For this review, take the finished solid that the model builds, in its own axes (mm). Face numbers are marked on the shaded views. Coordinates: 2 decimals unless noted, no trailing zeros.
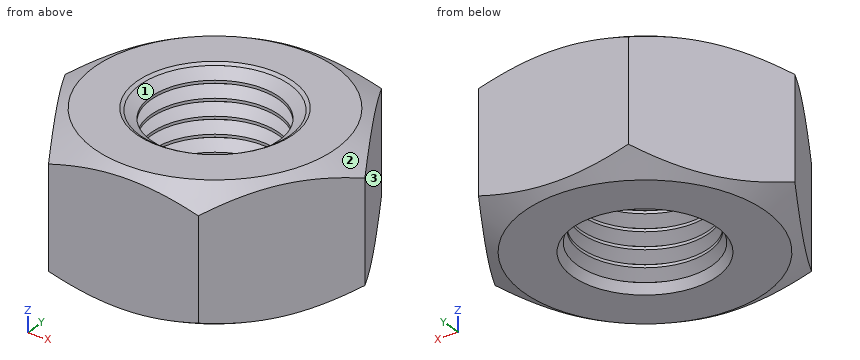
from build123d import *

# Parameters (mm, degrees)
SKETCH1_R               = 2.4585
BASENUT_DEPTH           = 5.2
ENDCHAMFER_SIZE         = 0.5415
ENDCHAMFER_SIZE2        = 0.312635171
ENDCHAMFER_PART_2_SIZE  = 0.5415
ENDCHAMFER_PART_2_SIZE2 = 0.312635171
LPATTERN10_COUNT        = 8
LPATTERN10_PITCH        = 0.6498


with BuildPart() as part:
    # Sketch1 → BaseNut (new body)
    with BuildSketch(Plane.XY):
        Polygon((5.773502692, 0), (2.886751346, 5), (-2.886751346, 5), (-5.773502692, 0), (-2.886751346, -5), (2.886751346, -5), align=None)
        Circle(SKETCH1_R, mode=Mode.SUBTRACT)
    extrude(amount=-BASENUT_DEPTH)

    # Sketch2 → Double-Chamfer (revolve, cut)
    with BuildSketch(Plane(origin=(0, 0, 0), x_dir=(1, 0, 0), z_dir=(0, 1, 0))):
        Polygon((-5.773502692, 5.2), (-4.625, 5.2), (-5.773502692, 4.536911662), align=None)
        Polygon((-5.773502692, 0.663088338), (-5.773502692, 0), (-4.625, 0), align=None)
    revolve(axis=Axis((0, 0, -3.375940562), (0, 0, 1)), mode=Mode.SUBTRACT)

    # EndChamfer
    endchamfer_edges = [part.edges().sort_by_distance(p)[0] for p in [
        (-2.4585, 0, -5.2),
    ]]
    endchamfer_side = [part.faces().sort_by_distance(p)[0] for p in [
        (-2.4585, 0, -2.6),
    ]]
    chamfer(endchamfer_edges, length=ENDCHAMFER_SIZE, length2=ENDCHAMFER_SIZE2, reference=endchamfer_side[0])

    # EndChamfer part 2
    endchamfer_part_2_edges = [part.edges().sort_by_distance(p)[0] for p in [
        (-2.4585, 0, 0),
    ]]
    endchamfer_part_2_side = [part.faces().sort_by_distance(p)[0] for p in [
        (4.494185245, 0, 0),
    ]]
    chamfer(endchamfer_part_2_edges, length=ENDCHAMFER_PART_2_SIZE, length2=ENDCHAMFER_PART_2_SIZE2, reference=endchamfer_part_2_side[0])

    # Sketch3 → Cut-Revolve10 (revolve, cut)
    with BuildSketch(Plane(origin=(0, 0, 0), x_dir=(1, 0, 0), z_dir=(0, 1, 0))):
        Polygon((-2.927452756, 4.6585), (-2.4585, 4.38775), (-1.917, 4.38775), (-1.917, 4.92925), (-2.4585, 4.92925), align=None)
    cut_revolve10 = revolve(axis=Axis((0, 0, -7.438254559), (0, 0, -1)), mode=Mode.SUBTRACT)

    # LPattern10: Cut-Revolve10 ×8
    with Locations(*[(0, 0, i * LPATTERN10_PITCH) for i in range(1, LPATTERN10_COUNT)]):
        add(cut_revolve10, mode=Mode.SUBTRACT)


solid = part.part
1. To check wall thickness, follow L1, parallel to Y at x = 0, z = -3; L2, parallel to X at y = 0.25, z = -5; L3, parallel to Y at x = 2, z = -2.4. State the ranges of each line that lie inside material, in increasing order.
Answer below:
L1: y = -5 to -2.46, 2.46 to 5
L2: x = -4.97 to -2.64, 2.64 to 4.97
L3: y = -5 to -1.43, 1.43 to 5
2. The part is to be moulded in two halves that separate along X. For the marked faces 1, 2 and 3, say which applies: +X half, -X half, draft (parallel to the pull), parting line (faces both ways), or undercut.
Answer below:
face 1: undercut
face 2: parting line
face 3: +X half
3. Clearance check with flat-ended pins moving along their axes: pin 1 Ø1 at (x, y) = (-2, -2) entering from +Z; pin 2 Ø5.5 at (x, y) = (0, 0) entering from +Z; pin 3 Ø2 at (y, z) = (-3.5, -4.5) entering from -X; pin 4 Ø2 at (y, z) = (2, -2.5) entering from +X. State where each tip first meets the part, or that it passes through.
Answer below:
pin 1: stops at z = 0
pin 2: stops at z = -0.21
pin 3: stops at x = -4.33
pin 4: stops at x = 5.2
